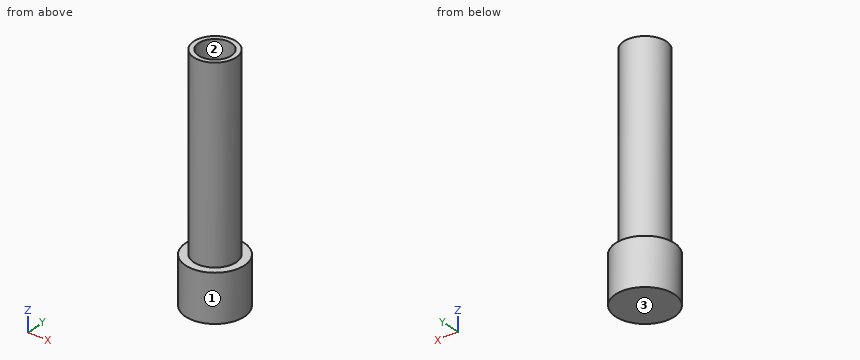
Autodesk Inventor part; units mm, degrees
ref_plane "YZ Plane" through (0, 0, 0) normal (1, 0, 0) x (0, 1, 0)
ref_plane "XZ Plane" through (0, 0, 0) normal (0, 1, 0) x (-1, 0, 0)
ref_plane "XY Plane" through (0, 0, 0) normal (0, 0, 1) x (1, 0, 0)
sketch "Esboço1" plane through (0, 0, 0) normal (0, 0, 1) x (1, 0, 0)
  circle A0 centre (0, 0) radius 0.9
  dimension "d0" = 1.8
extrude "Extrusão1" add sketch "Esboço1" against normal blind 10
sketch "Esboço2" plane through (0, 0, -10) normal (0, 0, -1) x (-1, 0, 0)
  circle A0 centre (0, 0) radius 1.25
  dimension "d3" = 2.5
extrude "Extrusão2" add sketch "Esboço2" against normal blind 2
sketch "Esboço3" plane through (0, 0, 0) normal (0, 0, 1) x (1, 0, 0)
  circle A0 centre (0, 0) radius 0.7
  dimension "d6" = 1.4
extrude "Extrusão3" cut sketch "Esboço3" against normal blind 8
thread "Rosca1"
properties material "Liga de Nickel-Copper 400"
Work out the finished part from the listing and answer in its coordinate system (mm). Face numbers are marked on the shaded views. Round coordinates to 2 decimals unless told otherwise and drop trailing zeros. Loops run counter-clockwise (first coordinate to the right, second up) from the corner with the lowest first, then second, coordinate; pieces in that order, holes last. Notation, with made-up numbers: (26.5, 76) - (30.5, 76) arc R25 cw to (30.5, 104) - close; hole circle Ø4 at (28.25, 82). An arc over 180 degrees is marked (long way). One line per item, written item: value.
Q1. Find section C-C on z = -2.25. Give the vertices of the cut face in (x, y).
Check values:
outline: circle Ø1.8 at (0, 0); hole circle Ø1.4 at (0, 0)
Q2. Find section D-D on y = -1.1. Give the vertices of the cut face in (x, z).
Check values:
outline: (-0.59, -10) - (0.59, -10) - (0.59, -8) - (-0.59, -8) - close
Q3. Straight lines are drawn through the part: probe 1 along Y at (x, z) = (0, -2.5); probe 2 along Z at (x, y) = (-0.7, 0.85); probe 3 along X at (y, z) = (0.35, -1.5). For each, find the intervals that lie inside material, in ascending order.
Check values:
probe 1: -0.9 to -0.7, 0.7 to 0.9
probe 2: -10 to -8
probe 3: -0.83 to -0.61, 0.61 to 0.83
Q4. Find section A-A on y = 0. Give the vertices of the cut face in (x, z), and give its area (3 significant figures).
Check values:
outline: (-1.25, -10) - (1.25, -10) - (1.25, -8) - (0.9, -8) - (0.9, 0) - (0.7, 0) - (0.7, -8) - (-0.7, -8) - (-0.7, 0) - (-0.9, 0) - (-0.9, -8) - (-1.25, -8) - close
area: 8.20 mm2
Q5. The mould has two halves that part along X. Classify the marked faces 1, 2 and 3: +X half, -X half, draft (parallel to the pull), parting line (faces both ways), or undercut.
Check values:
face 1: parting line
face 2: undercut
face 3: draft
Q6. This flat-tipped pin is pushed along its axis until it touches: pin 1 Ø1.5 at (x, z) = (-0.5, -3) entering from -Y. Where does it stop, or does it pass through?
Check values:
pin 1: y = -0.9
Q7. Find section B-B on x = -0.15. Give the vertices of the cut face in (y, z).
Check values:
outline: (-1.24, -10) - (1.24, -10) - (1.24, -8) - (0.89, -8) - (0.89, 0) - (0.68, 0) - (0.68, -8) - (-0.68, -8) - (-0.68, 0) - (-0.89, 0) - (-0.89, -8) - (-1.24, -8) - close
